For this review, take the finished solid that the model builds, in its own axes (mm). A direction names the side the tool comes from. Coordinates: 2 decimals unless noted, no trailing zeros. Write each loop counter-clockwise with the first axis right and the second up, starting at its lowest first coordinate (ties: lowest second). Pieces come first, ordered by that corner, then holes.
```python
from build123d import *

# Parameters (mm, degrees)
F0_R     = 67.5
F1_DEPTH = 25
F2_R     = 15
F2_W     = 45
F2_H     = 19.910383
F3_DEPTH = 7
F4_R     = 16


with BuildPart() as f1:
    # F0 (on Front) → F1 (new body)
    with BuildSketch(Plane.XZ):
        Circle(F0_R)
    extrude(amount=F1_DEPTH)

    # F2 (on Front) → F3 (join)
    with BuildSketch(Plane.XZ):
        with Locations((-23.179246, 21.990567)):
            Circle(F2_R)
        with Locations((21.820754, 21.990567)):
            Circle(F2_R)
        with Locations((-0.679246, -31.648587)):
            Rectangle(F2_W, F2_H)
    extrude(amount=-F3_DEPTH)

    # F4
    f4_edges = [f1.edges().sort_by_distance(p)[0] for p in [
        (21.820754, 3.5, -41.603778),
        (-23.179246, 3.5, -41.603778),
    ]]
    fillet(f4_edges, radius=F4_R)


solid = f1.part
```
1) Consider section B-B (z = -38). Give the boundary of the cut face in (x, y).
2) Consider section A-A (x = 0). Give the boundary of the cut face in (y, z), then the cut area to 3 significant figures.
3) Consider section C-C (y = -11). Give the boundary of the cut face in (x, z).
4) The part is to be moulded in two halves that separate along Z. For faces 5 (the face through (17.01, 3.55, -37.04)), 6 (the face through (21.821, 3, -24)), 7 (the face through (-15.12, 3.45, 34.64)), 8 (the face through (-1, 3, -21.693)), say which applies: pulls with the +Z half, pulls with the -Z half, needs draft (parallel to the pull), parting line crosses it, or undercut.
5) For L1, parallel to Y at x = -5.5, z = 47; L2, parallel to Z at x = -45.5, y = -11; L3, parallel to X at y = -16, z = -36, list the stretches that pass through material, from the lowest coordinate up.
6) Tool access review of faces 1 (the face through (36.128, 3.451, 26.496)), 2 (the face through (-53.57, -12.32, -41.07)), 3 (the face through (-23.179, 3, -24)), 4 (the face through (-1, 3, -41.604)): name each direction out of +Z, -Z, +X, -X, +Y, -Y from which nothing blocks a thin tool from reaching the whole face with its end or side.
7) Consider section D-D (z = 0). Give the boundary of the cut face in (x, y), then the cut area to 4 significant figures.
8) Clearance check with flat-ended pins moving along their axes: P1, Ø5.5, axis at x = 1, y = 2, coming from the -Z side; P2, Ø10, axis at x = 31, z = 0, coming from the +Y side; P3, Ø1.2, axis at y = 5, z = -23, coming from the -X side. State where each tip first meets the part, or that it passes through.
Results:
1. outline: (-55.79, -25) - (55.79, -25) - (55.79, 0) - (15.94, 0) - (15.94, 7) - (-17.3, 7) - (-17.3, 0) - (-55.79, 0) - close
2. outline: (-25, -67.5) - (0, -67.5) - (0, -41.6) - (7, -41.6) - (7, -21.69) - (0, -21.69) - (0, 67.5) - (-25, 67.5) - close
2. area: 3,510 mm2
3. outline: circle Ø135 at (0, 0)
4. face 5: pulls with the -Z half
4. face 6: needs draft
4. face 7: undercut
4. face 8: undercut
5. L1: y = -25 to 0
5. L2: z = -49.86 to 49.86
5. L3: x = -57.1 to 57.1
6. face 1: +Y
6. face 2: +Y, -Y
6. face 3: -Z, -X, +Y
6. face 4: -Z, +X, -X, +Y
7. outline: (-67.5, -25) - (67.5, -25) - (67.5, 0) - (-67.5, 0) - close
7. area: 3,375 mm2
8. P1: stops at z = -67.5
8. P2: stops at y = 0
8. P3: stops at x = -23.18
